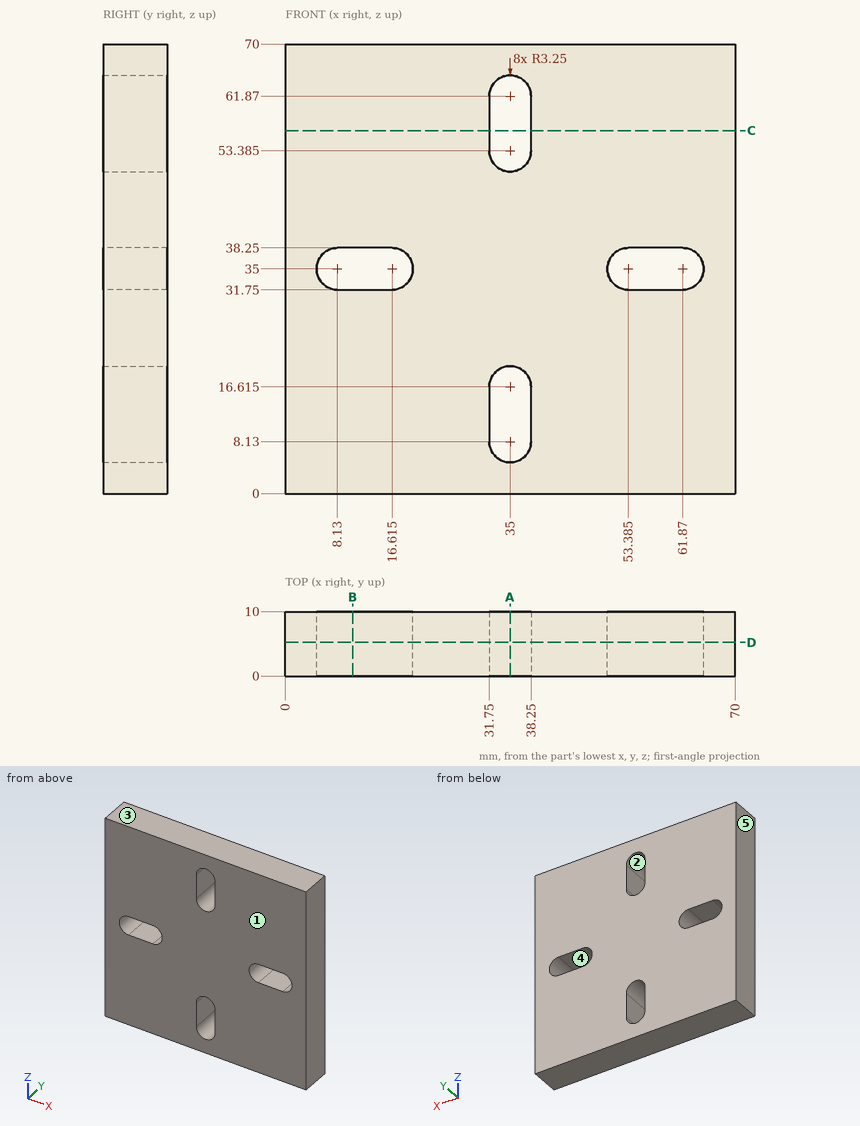
The figure shows three views and two pictorial views of one solid part (mm, origin at its lowest corner). Answer the questions. A direction names the side the tool comes from. Coordinates: 2 decimals unless noted, no trailing zeros. Order: outer loops, then holes, each group sorted by start corner. A loop starts at its lowest first (then second) coordinate and runs counter-clockwise, first axis right, second up.
Q1. A cutting plane is placed at D-D, the plane y = 5.25. State how many separate pieces and enclosed holes the cut face has, and give its area (3 significant figures).
Q2. A cutting plane is placed at A-A, the plane x = 35. Write down the section's boundary in (y, z) (1 decimal), and give its area (3 significant figures).
Q3. A cutting plane is placed at B-B, the plane x = 10.5. Write down the section's boundary in (y, z).
Q4. Consider line 1 (Z direction, x = 9, y = 1); line 2 (X direction, y = 8, z = 37). Determine where each line is inside the solid, lowest interval first.
Q5. For a pull along X with two mould halves and no side action, classify the marked faces 3, 4 and 5 as pulls with the +X half, pulls with the -X half, needs draft (parallel to the pull), parting line crosses it, or undercut.
Q6. A cutting plane is placed at C-C, the plane z = 56.5. Write down the section's boundary in (x, y).
Q7. Which of the six approach directions +Z, -Z, +X, -X, +Y, -Y give full straight-line access (tool end or side, diameter ignored) to the marked faces 1 and 2?
Answers follow:
1. separate pieces: 1
1. enclosed holes: 4
1. area: 4,550 mm2
2. outline: (0, 0) - (10, 0) - (10, 4.9) - (0, 4.9) - close; (0, 19.9) - (10, 19.9) - (10, 50.1) - (0, 50.1) - close; (0, 65.1) - (10, 65.1) - (10, 70) - (0, 70) - close
2. area: 400 mm2
3. outline: (0, 0) - (10, 0) - (10, 31.75) - (0, 31.75) - close; (0, 38.25) - (10, 38.25) - (10, 70) - (0, 70) - close
4. line 1: z = 0 to 31.75, 38.25 to 70
4. line 2: x = 0 to 5.57, 19.18 to 50.82, 64.43 to 70
5. face 3: needs draft
5. face 4: undercut
5. face 5: pulls with the -X half
6. outline: (0, 0) - (31.75, 0) - (31.75, 10) - (0, 10) - close; (38.25, 0) - (70, 0) - (70, 10) - (38.25, 10) - close
7. face 1: +Z, -Z, +X, -X, -Y
7. face 2: +Y, -Y
